from build123d import *

# Parameters (mm, degrees)
F0_R     = 8
F0_R_2   = 4.5
F0_R_3   = 3
F1_DEPTH = 5
F2_DEPTH = 10
F3_DEPTH = 7


with BuildPart() as f1:
    # F0 (on Front) → F1 (new body)
    with BuildSketch(Plane.XZ):
        Polygon((18.9996465826, 31.9180320948), (-17.4607320469, 31.9180320948), (-35.4878548533, 24.5556049049), (-48.3473874629, 18.9076156824), (-48.3473874629, -10.1699698716), (-16.3799077272, -21.7999331653), (-16.571868211, -48.7112030387), (9.7124404529, -48.7112030387), (20.7713786513, -35.5700962245), (29.6717043966, -20.5233637244), (29.840618372, -5.252843257), (29.1450880468, 13.5724376887), (23.4245508909, 23.8787811249), align=None)
        with Locations((0, -36)):
            Circle(F0_R, mode=Mode.SUBTRACT)
        with Locations((-38, 0)):
            Circle(F0_R, mode=Mode.SUBTRACT)
        with BuildLine():
            ThreePointArc((1.5, 9.8868599666), (7.0710678119, 7.0710678119), (9.8868599666, 1.5))
            Line((9.8868599666, 1.5), (24.8868599666, 1.5))
            Line((24.8868599666, 1.5), (24.8868599666, 0))
            Line((24.8868599666, 0), (24.8868599666, -1.5))
            Line((24.8868599666, -1.5), (9.8868599666, -1.5))
            ThreePointArc((9.8868599666, -1.5), (7.0710678119, -7.0710678119), (1.5, -9.8868599666))
            Line((1.5, -9.8868599666), (1.5, -24.8868599666))
            Line((1.5, -24.8868599666), (0, -24.8868599666))
            Line((0, -24.8868599666), (-1.5, -24.8868599666))
            Line((-1.5, -24.8868599666), (-1.5, -9.8868599666))
            ThreePointArc((-1.5, -9.8868599666), (-7.0710678119, -7.0710678119), (-9.8868599666, -1.5))
            Line((-9.8868599666, -1.5), (-24.8868599666, -1.5))
            Line((-24.8868599666, -1.5), (-24.8868599666, 0))
            Line((-24.8868599666, 0), (-24.8868599666, 1.5))
            Line((-24.8868599666, 1.5), (-9.8868599666, 1.5))
            ThreePointArc((-9.8868599666, 1.5), (-7.0710678119, 7.0710678119), (-1.5, 9.8868599666))
            Line((-1.5, 9.8868599666), (-1.5, 24.8868599666))
            Line((-1.5, 24.8868599666), (0, 24.8868599666))
            Line((0, 24.8868599666), (1.5, 24.8868599666))
            Line((1.5, 24.8868599666), (1.5, 9.8868599666))
        make_face(mode=Mode.SUBTRACT)
        with BuildLine():
            ThreePointArc((9.8868599666, -1.5), (9.971674876, -0.7521304187), (10, 0))
            ThreePointArc((10, 0), (9.971674876, 0.7521304187), (9.8868599666, 1.5))
            ThreePointArc((9.8868599666, 1.5), (7.0710678119, 7.0710678119), (1.5, 9.8868599666))
            ThreePointArc((1.5, 9.8868599666), (0, 10), (-1.5, 9.8868599666))
            ThreePointArc((-1.5, 9.8868599666), (-7.0710678119, 7.0710678119), (-9.8868599666, 1.5))
            ThreePointArc((-9.8868599666, 1.5), (-10, 0), (-9.8868599666, -1.5))
            ThreePointArc((-9.8868599666, -1.5), (-7.0710678119, -7.0710678119), (-1.5, -9.8868599666))
            ThreePointArc((-1.5, -9.8868599666), (0, -10), (1.5, -9.8868599666))
            ThreePointArc((1.5, -9.8868599666), (7.0710678119, -7.0710678119), (9.8868599666, -1.5))
        make_face()
        Circle(F0_R_2, mode=Mode.SUBTRACT)
        with Locations((-38, 0)):
            Circle(F0_R)
        with Locations((-38, 0)):
            Circle(F0_R_3, mode=Mode.SUBTRACT)
        with Locations((0, -36)):
            Circle(F0_R)
        with Locations((0, -36)):
            Circle(F0_R_3, mode=Mode.SUBTRACT)
        with BuildLine():
            ThreePointArc((-9.8868599666, -1.5), (-10, 0), (-9.8868599666, 1.5))
            Line((-9.8868599666, 1.5), (-24.8868599666, 1.5))
            Line((-24.8868599666, 1.5), (-24.8868599666, 0))
            Line((-24.8868599666, 0), (-24.8868599666, -1.5))
            Line((-24.8868599666, -1.5), (-9.8868599666, -1.5))
        make_face()
        with BuildLine():
            ThreePointArc((-1.5, 9.8868599666), (0, 10), (1.5, 9.8868599666))
            Line((1.5, 9.8868599666), (1.5, 24.8868599666))
            Line((1.5, 24.8868599666), (0, 24.8868599666))
            Line((0, 24.8868599666), (-1.5, 24.8868599666))
            Line((-1.5, 24.8868599666), (-1.5, 9.8868599666))
        make_face()
        with BuildLine():
            ThreePointArc((9.8868599666, 1.5), (9.971674876, 0.7521304187), (10, 0))
            ThreePointArc((10, 0), (9.971674876, -0.7521304187), (9.8868599666, -1.5))
            Line((9.8868599666, -1.5), (24.8868599666, -1.5))
            Line((24.8868599666, -1.5), (24.8868599666, 0))
            Line((24.8868599666, 0), (24.8868599666, 1.5))
            Line((24.8868599666, 1.5), (9.8868599666, 1.5))
        make_face()
        with BuildLine():
            Line((1.5, -24.8868599666), (1.5, -9.8868599666))
            ThreePointArc((1.5, -9.8868599666), (0, -10), (-1.5, -9.8868599666))
            Line((-1.5, -9.8868599666), (-1.5, -24.8868599666))
            Line((-1.5, -24.8868599666), (0, -24.8868599666))
            Line((0, -24.8868599666), (1.5, -24.8868599666))
        make_face()
    extrude(amount=-F1_DEPTH)

    # F0 (on Front) → F2 (join)
    with BuildSketch(Plane.XZ):
        with BuildLine():
            ThreePointArc((9.8868599666, -1.5), (9.971674876, -0.7521304187), (10, 0))
            ThreePointArc((10, 0), (9.971674876, 0.7521304187), (9.8868599666, 1.5))
            ThreePointArc((9.8868599666, 1.5), (7.0710678119, 7.0710678119), (1.5, 9.8868599666))
            ThreePointArc((1.5, 9.8868599666), (0, 10), (-1.5, 9.8868599666))
            ThreePointArc((-1.5, 9.8868599666), (-7.0710678119, 7.0710678119), (-9.8868599666, 1.5))
            ThreePointArc((-9.8868599666, 1.5), (-10, 0), (-9.8868599666, -1.5))
            ThreePointArc((-9.8868599666, -1.5), (-7.0710678119, -7.0710678119), (-1.5, -9.8868599666))
            ThreePointArc((-1.5, -9.8868599666), (0, -10), (1.5, -9.8868599666))
            ThreePointArc((1.5, -9.8868599666), (7.0710678119, -7.0710678119), (9.8868599666, -1.5))
        make_face()
        Circle(F0_R_2, mode=Mode.SUBTRACT)
        with Locations((0, -36)):
            Circle(F0_R)
        with Locations((0, -36)):
            Circle(F0_R_3, mode=Mode.SUBTRACT)
        with Locations((-38, 0)):
            Circle(F0_R)
        with Locations((-38, 0)):
            Circle(F0_R_3, mode=Mode.SUBTRACT)
    extrude(amount=-F2_DEPTH)

    # F0 (on Front) → F3 (join)
    with BuildSketch(Plane.XZ):
        with BuildLine():
            ThreePointArc((-9.8868599666, -1.5), (-10, 0), (-9.8868599666, 1.5))
            Line((-9.8868599666, 1.5), (-24.8868599666, 1.5))
            Line((-24.8868599666, 1.5), (-24.8868599666, 0))
            Line((-24.8868599666, 0), (-24.8868599666, -1.5))
            Line((-24.8868599666, -1.5), (-9.8868599666, -1.5))
        make_face()
        with BuildLine():
            Line((1.5, -24.8868599666), (1.5, -9.8868599666))
            ThreePointArc((1.5, -9.8868599666), (0, -10), (-1.5, -9.8868599666))
            Line((-1.5, -9.8868599666), (-1.5, -24.8868599666))
            Line((-1.5, -24.8868599666), (0, -24.8868599666))
            Line((0, -24.8868599666), (1.5, -24.8868599666))
        make_face()
        with BuildLine():
            ThreePointArc((9.8868599666, 1.5), (9.971674876, 0.7521304187), (10, 0))
            ThreePointArc((10, 0), (9.971674876, -0.7521304187), (9.8868599666, -1.5))
            Line((9.8868599666, -1.5), (24.8868599666, -1.5))
            Line((24.8868599666, -1.5), (24.8868599666, 0))
            Line((24.8868599666, 0), (24.8868599666, 1.5))
            Line((24.8868599666, 1.5), (9.8868599666, 1.5))
        make_face()
        with BuildLine():
            ThreePointArc((-1.5, 9.8868599666), (0, 10), (1.5, 9.8868599666))
            Line((1.5, 9.8868599666), (1.5, 24.8868599666))
            Line((1.5, 24.8868599666), (0, 24.8868599666))
            Line((0, 24.8868599666), (-1.5, 24.8868599666))
            Line((-1.5, 24.8868599666), (-1.5, 9.8868599666))
        make_face()
    extrude(amount=-F3_DEPTH)

    # F5 (on Top) → F6 (revolve, cut)
    with BuildSketch(Plane.XY):
        with BuildLine():
            ThreePointArc((-38, 9.9469926208), (-41.7, 6.2469926208), (-38, 2.5469926208))
            Line((-38, 2.5469926208), (-38, 9.9469926208))
        make_face()
    revolve(axis=Axis((-38, 4.9734963104, 0), (0, -1, 0)), mode=Mode.SUBTRACT)

    # F4 (on Right) → F7 (revolve, cut)
    with BuildSketch(Plane.YZ):
        with BuildLine():
            Line((2.9804437381, -35.9969779618), (10.3804399341, -35.9894746928))
            ThreePointArc((10.3804399341, -35.9894746928), (6.6766902016, -32.2932282293), (2.9804437381, -35.9969779618))
        make_face()
    revolve(axis=Axis((0, 3.1299426986, -35.9968263765), (0, 0.9999994859, 0.0010139553)), mode=Mode.SUBTRACT)

    # F4 (on Right) → F8 (revolve, cut)
    with BuildSketch(Plane.YZ):
        with BuildLine():
            Line((0, 0), (10, 0))
            ThreePointArc((10, 0), (5, 6.1049875621), (0, 0))
        make_face()
    revolve(axis=Axis((0, 5, 0), (0, -1, 0)), mode=Mode.SUBTRACT)


solid = f1.part
Check sheet for the modelled part. Datum: model origin and axes. Units: mm. A direction names the side the tool comes from. Give positions to 0.01 mm unless a question says otherwise; leave off trailing zeros. Loops run counter-clockwise (first coordinate to the right, second up) from the corner with the lowest first, then second, coordinate; pieces in that order, holes last. Notation, with made-up numbers: M 87.5,-7 L 112.5,-7 A25 ccw 112.5,19 Z; hole C -14,11 d11. An arc over 180 degrees is marked long. Answer as a JSON object with one key per item and string values. Group by question number.
Q1. Access from +Z, -Z, +X, -X, +Y, -Y to the whole of each face (thin tool, end or side, straight path). Record for faces 1 (the flat face through (0, 6, -24.887)), 2 (the flat face through (-17, 6, 1.5)), 3 (the flat face through (-24.887, 6, 0)).
Q2. Cross-section at C-C on z = 20. Record the cut outline in (x, y).
Q3. Release check for a two-part mould opening along Z. For faces 4 (the cylindrical face through (-1.041, 7.465, -28.068)), 5 (the flat face through (-17, 6, -1.5)), 6 (the flat face through (3.4, 10, -35.9)) record: released by +Z, released by -Z, zero draft, split by the parting line, or undercut.
Q4. Cross-section at B-B on x = 0. Give the number of separate pieces and of enclosed holes in the cut face, then the cut area to 3 significant figures.
Q5. Material ranges on line 1 along X through (y, z) = (1.7, 0); line 2 along X through (y, z) = (0.35, 0); line 3 along Y through (x, z) = (17, 19.5), recorded low to high. Write a range as [from, to].
Q6. Cross-section at D-D on x = 14. Record the cut outline in (y, z), then the cut area to 3 significant figures.
Q7. Cross-section at A-A on x = -38. Record the cut outline in (y, z), then the cut area to 3 significant figures.
Q8. Go/stop test with flat-tipped pins: P1, Ø1.5, axis at x = -28, y = 4, coming from the -Z side; P2, Ø1, axis at x = -19, y = 6.5, coming from the -Z side; P3, Ø8, axis at x = -19, z = 4, coming from the +Y side. Record where each tip stops, or that it passes through.
Evaluation:
{
 "1": {"face 1": "+X, -X, +Y", "face 2": "+Z, +Y", "face 3": "+Z, -Z, +Y"},
 "2": {"outline": "M -45.86,0 L 25.58,0 L 25.58,5 L 1.5,5 L 1.5,7 L -1.5,7 L -1.5,5 L -45.86,5 Z"},
 "3": {"face 4": "undercut", "face 5": "released by -Z", "face 6": "zero draft"},
 "4": {"separate pieces": "3", "enclosed holes": "0", "area": "472 mm2"},
 "5": {"line 1": "x = [-48.35, -41], [-35, -4.89], [4.89, 29.65]", "line 2": "x = [-48.35, -41], [-35, -4.5], [4.5, 29.65]", "line 3": "y = [0, 5]"},
 "6": {"outline": "M 0,-43.62 L 5,-43.62 L 5,-1.5 L 7,-1.5 L 7,1.5 L 5,1.5 L 5,31.92 L 0,31.92 Z", "area": "384 mm2"},
 "7": {"outline": "M 0,-13.93 L 5,-13.93 L 5,-8 L 10,-8 L 10,-3 L 8.41,-3 A3.7 cw 4.08,-3 L 0,-3 Z; M 0,3 L 4.08,3 A3.7 cw 8.41,3 L 10,3 L 10,8 L 5,8 L 5,23.45 L 0,23.45 Z", "area": "203 mm2"},
 "8": {"P1": "stops at z = -17.85", "P2": "stops at z = -1.5", "P3": "stops at y = 7"}
}
